Model file for the job. Use its own axes, mm. Face numbers are marked on the shaded views. A direction names the side the tool comes from. Round coordinates to 2 decimals unless told otherwise and drop trailing zeros. Order: outer loops, then holes, each group sorted by start corner. A loop starts at its lowest first (then second) coordinate and runs counter-clockwise, first axis right, second up. Notation, with made-up numbers: (-6, 51.25) -> (39, 51.25) arc R15 ccw to (39, 75.25) -> close; hole circle Ø10 at (43.5, 64). An arc over 180 degrees is marked (long way). Answer as CSV lines item,"result".
```python
from build123d import *

# Parameters (mm, degrees)
SKETCH1_W           = 6.5
SKETCH1_H           = 25
BOSS_EXTRUDE1_DEPTH = 40
SKETCH2_R           = 1.25
CUT_EXTRUDE1_DEPTH  = 10
SKETCH3_R           = 9
BOSS_EXTRUDE2_DEPTH = 67.9


with BuildPart() as part:
    # Sketch1 → Boss-Extrude1 (new body)
    with BuildSketch(Plane.XY):
        with Locations((-36.95, -62.9)):
            Rectangle(SKETCH1_W, SKETCH1_H)
    boss_extrude1 = extrude(amount=BOSS_EXTRUDE1_DEPTH)

    # Sketch2 → Cut-Extrude1 (cut)
    with BuildSketch(Plane(origin=(0, 0, 0), x_dir=(-1, 0, 0), z_dir=(0, 0, -1))):
        with Locations((37.2, -55.4)):
            Circle(SKETCH2_R)
        with Locations((37.2, -64)):
            Circle(SKETCH2_R)
    cut_extrude1 = extrude(amount=-CUT_EXTRUDE1_DEPTH, mode=Mode.SUBTRACT)

    # Sketch3 → Boss-Extrude2 (add)
    with BuildSketch(Plane(origin=(-33.7, 0, 0), x_dir=(0, 0, -1), z_dir=(1, 0, 0))):
        with Locations(Location((-29, -66.4, 0), (0, 0, 180))):
            Circle(SKETCH3_R)
    extrude(amount=BOSS_EXTRUDE2_DEPTH)

    # Mirror1: Boss-Extrude1, Cut-Extrude1 across plane
    add(boss_extrude1.mirror(Plane(origin=(0.25, 0, 0), x_dir=(0, 0, 1), z_dir=(1, 0, 0))))
    add(cut_extrude1.mirror(Plane(origin=(0.25, 0, 0), x_dir=(0, 0, 1), z_dir=(1, 0, 0))), mode=Mode.SUBTRACT)


solid = part.part
```
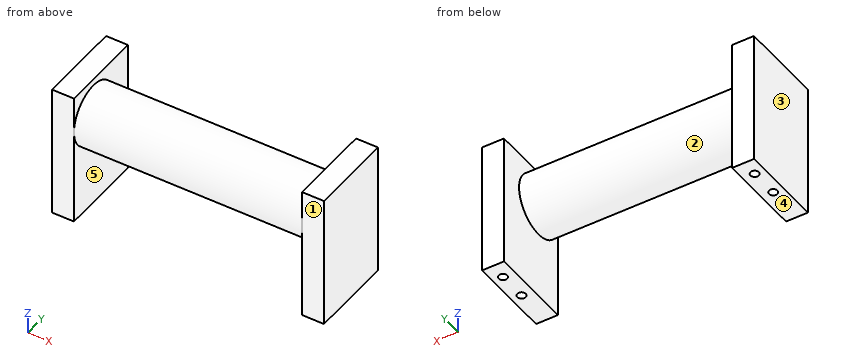
Q1. Saw through at D-D (z = 31). Write the cut outline in (x, y).
Checks:
outline,"(-40.2, -75.4) -> (-33.7, -75.4) -> (-33.7, -75.17) -> (34.2, -75.17) -> (34.2, -75.4) -> (40.7, -75.4) -> (40.7, -50.4) -> (34.2, -50.4) -> (34.2, -57.63) -> (-33.7, -57.63) -> (-33.7, -50.4) -> (-40.2, -50.4) -> close"
Q2. Saw through at C-C (x = 37.7). Write the cut outline in (y, z).
Checks:
outline,"(-75.4, 0) -> (-65.25, 0) -> (-65.25, 10) -> (-62.75, 10) -> (-62.75, 0) -> (-56.65, 0) -> (-56.65, 10) -> (-54.15, 10) -> (-54.15, 0) -> (-50.4, 0) -> (-50.4, 40) -> (-75.4, 40) -> close"
Q3. Tool access for the marked faces 1 and 2: list every direction of +Z, -Z, +X, -X, +Y, -Y with a clear straight run to the whole face (end or side of a thin tool).
Checks:
face 1,"+Z, -Z, +X, -X, -Y"
face 2,"none"
Q4. Mould opens along X. For the marked faces 3, 4 and 5 say: +X half, -X half, draft (parallel to the pull), parting line (faces both ways), or undercut.
Checks:
face 3,"-X half"
face 4,"draft"
face 5,"undercut"
Q5. Saw through at A-A (z = 13). Write the cut outline in (x, y).
Checks:
outline,"(-40.2, -75.4) -> (-33.7, -75.4) -> (-33.7, -50.4) -> (-40.2, -50.4) -> close; (34.2, -75.4) -> (40.7, -75.4) -> (40.7, -50.4) -> (34.2, -50.4) -> close"
Q6. Saw through at B-B (y = -55.4). Write the cut outline in (x, z), plus the area to 3 significant figures.
Checks:
outline,"(-40.2, 0) -> (-38.45, 0) -> (-38.45, 10) -> (-35.95, 10) -> (-35.95, 0) -> (-33.7, 0) -> (-33.7, 40) -> (-40.2, 40) -> close; (34.2, 0) -> (36.45, 0) -> (36.45, 10) -> (38.95, 10) -> (38.95, 0) -> (40.7, 0) -> (40.7, 40) -> (34.2, 40) -> close"
area,"470 mm²"
Q7. Flat gauge pins, fed straight in: pin 1 (0.8 mm diameter, centred on x = 38, y = -63.5, fed in from -Z); pin 2 (10 mm diameter, centred on x = 15, z = 35.5, fed in from +Y); pin 3 (8 mm diameter, centred on x = -5.5, z = 36, fed in from -Y). Where does each tip first touch, or does it go through?
Checks:
pin 1,"z = 10"
pin 2,"y = -57.53"
pin 3,"y = -74.89"
Q8. Wall check: L1, parallel to Y at x = -37.2, z = 5.75; L2, parallel to X at y = -53, z = 7; L3, parallel to Y at x = 37, z = 2. Give the ranges that are in metal, low to high. Write a range as [from, to].
Checks:
L1,"[-75.4, -65.25], [-62.75, -56.65], [-54.15, -50.4]"
L2,"[-40.2, -33.7], [34.2, 40.7]"
L3,"[-75.4, -65.04], [-62.96, -56.44], [-54.36, -50.4]"
